Geometry check sheet. Reference: the model listing, model coordinates, mm. A direction names the side the tool comes from. Round coordinates to 2 decimals unless told otherwise and drop trailing zeros. Write each loop counter-clockwise with the first axis right and the second up, starting at its lowest first coordinate (ties: lowest second). Pieces come first, ordered by that corner, then holes. Notation, with made-up numbers: M -13.5,17.25 L 24.5,17.25 A19 cw 24.5,46.25 Z; hole C 38,23.25 d10. An arc over 180 degrees is marked long. Answer as CSV lines item,"result". Start each with the question number.
Autodesk Inventor part; units mm, degrees
ref_plane "YZ Plane" through (0, 0, 0) normal (1, 0, 0) x (0, 1, 0)
ref_plane "XZ Plane" through (0, 0, 0) normal (0, 1, 0) x (-1, 0, 0)
ref_plane "XY Plane" through (0, 0, 0) normal (0, 0, 1) x (1, 0, 0)
sketch "Sketch1" plane through (0, 0, 0) normal (0, 1, 0) x (-1, 0, 0)
  circle A0 centre (0, 0) radius 12.5
  dimension "d0" = 25
extrude "Extrusion1" add sketch "Sketch1" along normal blind 27
sketch "Sketch2" plane through (0, 27, 0) normal (0, 1, 0) x (1, 0, 0)
  circle A0 centre (0, 0) radius 7.5
  arc A1 (-1, -2.8284) -> (-1, 2.8284) centre (0, 0) ccw
  line L0 (3, 0) -> (-1, 0) construction
  line L1 (-1, 0) -> (-1, 2.8284) construction
  line L2 (-1, 2.8284) -> (-1, -2.8284)
  dimension "d4" = 15
  dimension "d5" = 6
  dimension "d6" = 4
extrude "Extrusion2" add sketch "Sketch2" along normal blind 5
sketch "Sketch3" plane through (0, 0, 0) normal (0, -1, 0) x (1, 0, 0)
  circle A0 centre (0, 0) radius 5.25
  dimension "d9" = 10.5
extrude "Extrusion3" cut sketch "Sketch3" against normal blind 25
sketch "Sketch6" plane through (0, 0, 0) normal (0, 0, 1) x (1, 0, 0)
  line L0 (0, 12.9265) -> (-19.9756, 12.9265) construction
  line L1 (0, 12.9265) -> (20.0738, 12.9265) construction
  line L2 (0, 0) -> (0, 12.9) construction
  dimension "d19" = 12.9
ref_plane "Work Plane1" through (-19.9756, 12.9265, 0) normal (-1, 0, 0) x (0, -1, 0)
sketch "Sketch7" plane through (-19.9756, 12.9265, 0) normal (-1, 0, 0) x (0, -1, 0)
  circle A0 centre (0, 0) radius 4
  point P0 (12.9265, 0)
  dimension "d16" = 8
extrude "Extrusion5" cut sketch "Sketch7" against normal blind 10
ref_plane "Work Plane2" through (20.0738, 12.9265, 0) normal (1, 0, 0) x (0, 1, 0)
sketch "Sketch8" plane through (20.0738, 12.9265, 0) normal (1, 0, 0) x (0, 1, 0)
  line L0 (-3.5, -2.0207) -> (-3.5, 2.0207)
  line L1 (-3.5, 2.0207) -> (0, 4.0415)
  line L2 (0, 4.0415) -> (3.5, 2.0207)
  line L3 (3.5, 2.0207) -> (3.5, -2.0207)
  line L4 (3.5, -2.0207) -> (0, -4.0415)
  line L5 (0, -4.0415) -> (-3.5, -2.0207)
  point P0 (-12.9265, 0)
  point P1 (0, 0)
extrude "Extrusion6" cut sketch "Sketch8" against normal blind 17.9375
sketch "Sketch9" plane through (-19.9756, 12.9265, 0) normal (-1, 0, 0) x (0, -1, 0)
  circle A0 centre (0, 0) radius 2.25
  point P0 (12.9265, 0)
  dimension "d22" = 4.5
extrude "Extrusion7" cut sketch "Sketch9" against normal blind 17.9375
properties part number "StuurPotentiometerConnector3.0"
1) Section check C-C, the plane y = 4.5. Record the cut outline in (x, z).
2) Section check D-D, the plane x = 0. Record the cut outline in (y, z), plus the area to 4 significant figures.
3) Mould release check, pull along X, two halves, no side actions. Record for faces 1 (the cylindrical face through (-7.493, 29.465, 0.33)), 2 (the flat face through (-9.976, 11, -2)), 3 (the cylindrical face through (3, 29, 0)), 4 (the flat face through (7.906, 14.701, -3.017)): released by +X, released by -X, zero draft, split by the parting line, or undercut.
4) Section check B-B, the plane x = 5.75. Record the cut outline in (y, z), plus the area to 3 significant figures.
5) Scan lines: line 1 (Z direction, x = 0, y = 17.5); line 2 (Y direction, x = -5.9, z = 0); line 3 (Y direction, x = -8.55, z = 0). Record each from-to range of solid material in increasing order. Write a range as from..to.
6) Section check A-A, the plane z = 0. Record the cut outline in (x, y).
7) Go/stop test with flat-tipped pins: pin 1 (10 mm diameter, centred on x = -6, z = -7, fed in from +Y); pin 2 (6 mm diameter, centred on y = 12.93, z = 0, fed in from -X); pin 3 (5 mm diameter, centred on x = -7, y = 9, fed in from -Z); pin 4 (1.5 mm diameter, centred on y = 29.5, z = 1.5, fed in from +X). Record where each tip stops, or that it passes through.
8) Access from +Z, -Z, +X, -X, +Y, -Y to the whole of each face (thin tool, end or side, straight path). Record for faces 5 (the flat face through (0, 25, 0)), 6 (the flat face through (1, 27, 0)), 7 (the flat face through (9, 9.426, 0)), 8 (the cylindrical face through (-10.97, 9.23, -1.53)).
Results:
1,outline,"C 0,0 d25; hole C 0,0 d10.5"
2,outline,"M 0,-12.5 L 27,-12.5 L 27,-7.5 L 32,-7.5 L 32,-3 L 27,-3 L 27,3 L 32,3 L 32,7.5 L 27,7.5 L 27,12.5 L 0,12.5 L 0,5.25 L 25,5.25 L 25,-5.25 L 0,-5.25 Z"
2,area,"457.5 mm^2"
3,face 1,"split by the parting line"
3,face 2,"released by -X"
3,face 3,"undercut"
3,face 4,"zero draft"
4,outline,"M 0,-11.1 L 27,-11.1 L 27,-4.82 L 32,-4.82 L 32,4.82 L 27,4.82 L 27,11.1 L 0,11.1 Z; hole M 9.43,-2.02 L 12.93,-4.04 L 16.43,-2.02 L 16.43,2.02 L 12.93,4.04 L 9.43,2.02 Z"
4,area,"605 mm^2"
5,line 1,"z = -12.5..-5.25, 5.25..12.5"
5,line 2,"y = 0..10.68, 15.18..32"
5,line 3,"y = 0..10.68, 15.18..27"
6,outline,"M -12.5,0 L -5.25,0 L -5.25,10.68 L -9.98,10.68 L -9.98,8.93 L -12.5,8.93 Z; M -12.5,16.93 L -9.98,16.93 L -9.98,15.18 L -5.25,15.18 L -5.25,25 L 5.25,25 L 5.25,16.43 L 12.5,16.43 L 12.5,27 L 7.5,27 L 7.5,32 L 3,32 L 3,27 L -1,27 L -1,32 L -7.5,32 L -7.5,27 L -12.5,27 Z; M 5.25,0 L 12.5,0 L 12.5,9.43 L 5.25,9.43 Z"
7,pin 1,"stops at y = 32"
7,pin 2,"stops at x = -9.98"
7,pin 3,"stops at z = -11.66"
7,pin 4,"stops at x = 7.46"
8,face 5,"-Y"
8,face 6,"+Y"
8,face 7,"+X"
8,face 8,"-X"
